The listing builds one solid part. Answer for the finished solid, in the listing's coordinates (mm). A direction names the side the tool comes from. Coordinates: 2 decimals unless noted, no trailing zeros. Order: outer loops, then holes, each group sorted by start corner. A loop starts at its lowest first (then second) coordinate and runs counter-clockwise, first axis right, second up. Notation, with made-up numbers: (77.25, 43) -> (126.25, 43) arc R31 ccw to (126.25, 80) -> close; hole circle Ø9 at (56, 39). An arc over 180 degrees is marked (long way). Answer in a Markdown table with one row per item. Add a question column.
Solid Edge part; units mm, degrees
sketch "Sketch1" plane through (0, 0, 0) normal (1, 0, 0) x (0, 1, 0)
  circle A0 centre (0, 0) radius 3
extrude "Protrusion1" add sketch "Sketch1" along normal mid plane 46
chamfer "Chamfer_1" distance 0.5 angle 45 1 edges at (23, -3, 0)
chamfer "Chamfer_2" distance 0.5 angle 45 1 edges at (-23, -3, 0)
sketch "Sketch2" plane through (23, 0, 0) normal (1, 0, 0) x (0, 1, 0)
  line L0 (-2.2361, 3.1915) -> (2.2361, 3.1915)
  line L1 (2.2361, 3.1915) -> (2.2361, 2)
  line L2 (0, 2) -> (2.2361, 2)
  line L3 (0, 2) -> (-2.2361, 2)
  line L4 (-2.2361, 2) -> (-2.2361, 3.1915)
extrude "ExtrudedCutout_1" cut sketch "Sketch2" along normal mid plane 6
mirror "Mirror1" about plane through (0, 0, 0) normal (1, 0, 0) of "ExtrudedCutout_1"
properties material "PVC"
Q1. A cutting plane is placed at A-A (y = 0). Determine the outline of the cut face in (x, z), then the cut area to 3 significant figures.
Q2. A cutting plane is placed at C-C (z = 2.6). Determine the outline of the cut face in (x, y).
Q3. Straight lines are drawn through the part: line 1 (Y direction, x = 2.5, z = -0.1); line 2 (X direction, y = -1.45, z = 2.3); line 3 (Z direction, x = 2, y = 0.6). For each, find the intervals that lie inside material, in ascending order.
Q4. For faces 1 (the face through (-20, 0, 2.4)), 2 (the face through (20, 0, 2.4)), 3 (the face through (0.32, -0.65, -2.93)), determine the directions among +Z, -Z, +X, -X, +Y, -Y from which every point of the face is accessible in a straight line to the end or side of a thin tool.
Q5. A cutting plane is placed at B-B (x = -7). Determine the outline of the cut face in (y, z), then the cut area to 3 significant figures.
Q6. Given pin 1 (1.5 mm diameter, centred on x = 6.5, y = 2, fed in from -Z); pin 2 (1.5 mm diameter, centred on x = 21, y = -1, fed in from +Z); pin 3 (0.5 mm diameter, centred on y = -0.5, z = 2.5, fed in from -X), each flat-ended and moving along its own axis, determine where each tip first touches the part or whether it passes through.
Returned:
| question | item | result |
|---|---|---|
| 1 | outline | (-23, -2.5) -> (-22.5, -3) -> (22.5, -3) -> (23, -2.5) -> (23, 2) -> (20, 2) -> (20, 3) -> (-20, 3) -> (-20, 2) -> (-23, 2) -> close |
| 1 | area | 270 mm² |
| 2 | outline | (-20, -1.5) -> (20, -1.5) -> (20, 1.5) -> (-20, 1.5) -> close |
| 3 | line 1 | y = -3 to 3 |
| 3 | line 2 | x = -20 to 20 |
| 3 | line 3 | z = -2.94 to 2.94 |
| 4 | face 1 | +Z, -X, +Y, -Y |
| 4 | face 2 | +Z, +X, +Y, -Y |
| 4 | face 3 | +X, -X |
| 5 | outline | circle Ø6 at (0, 0) |
| 5 | area | 28.3 mm² |
| 6 | pin 1 | stops at z = -2.73 |
| 6 | pin 2 | stops at z = 2 |
| 6 | pin 3 | stops at x = -20 |
